Input: part model. Units: mm. Frame: model coordinates. A direction names the side the tool comes from. Coordinates: 2 decimals unless noted, no trailing zeros. Write each loop counter-clockwise with the first axis right and the second up, starting at its lowest first coordinate (ties: lowest second). Pieces come first, ordered by that corner, then holes. Notation, with made-up numbers: (4.5, 54) -> (54.5, 54) arc R21 ccw to (54.5, 63) -> close; hole circle Ø11 at (69.5, 22). An arc over 180 degrees is marked (long way). Use one line per item in the form item = value. Start each with the question number.
(1) Ray query, line 1 along X through (y, z) = (1.5, 0); line 2 along X through (y, z) = (1.5, -55.5); line 3 along Z through (x, y) = (-34.5, 0.5). Return the intervals inside material, ascending.
(2) Cut plane C-C on x = -56. Return the cut outline in (y, z).
(3) First-contact query: pin 1 (1.2 mm diameter, centred on y = 5, z = 0, fed in from +X); pin 2 (2 mm diameter, centred on y = 6, z = -0.5, fed in from -X); pin 3 (1.5 mm diameter, centred on x = -25.5, z = 39.5, fed in from -Y); pin 4 (1.5 mm diameter, centred on y = 9, z = -10, fed in from -X). Flat tips, straight axial feed; report the tip coordinate or a pass-through.
(4) Cut plane D-D on z = -26. Return the cut outline in (x, y) (3 decimals), plus the area to 3 significant figures.
(5) Cut plane B-B on y = 4.75. State how many separate pieces and enclosed holes the cut face has, plus the area to 3 significant figures.
(6) Cut plane A-A on z = -11. Return the cut outline in (x, y) (3 decimals).
(7) Pull-direction query (X, two-part tool) for faces 1 (the face through (62.101, 6, 0)), 2 (the face through (22.38, 4.93, 71.06)), 3 (the face through (-16, 0, 32)); classes: released by +X, released by -X, zero draft, split by the parting line, or undercut.
(8) Set-up query: faces 4 (the face through (65.701, 6, 0)), 5 (the face through (-30.078, 8.479, 51.137)). Return all of +Z, -Z, +X, -X, +Y, -Y with unobstructed straight access to the full face (end or side cutting, diameter ignored); none if empty.
```python
from build123d import *

# Parameters (mm, degrees)
CROQUIS1_R                                     = 74.5
CROQUIS1_R_2                                   = 33
SALIENTE_EXTRUIR1_DEPTH                        = 7
CROQUIS2_R                                     = 74.5
SALIENTE_EXTRUIR2_DEPTH                        = 3
CROQUIS4_R                                     = 2.5
CORTAR_EXTRUIR2_DEPTH                          = 106.832414694
CSK_START                                      = -1
CSK_SLOT_FOR_M3_FLAT_HEAD_MACHINE_SCREW2_DEPTH = 12
CIRPATTERN1_COUNT                              = 6


with BuildPart() as part:
    # Croquis1 → Saliente-Extruir1 (new body)
    with BuildSketch(Plane(origin=(0, 0, 0), x_dir=(1, 0, 0), z_dir=(0, 1, 0))):
        with Locations(Location((0, 0, 0), (0, 0, 270))):
            Circle(CROQUIS1_R)
        with Locations(Location((0, 0, 0), (0, 0, 270))):
            Circle(CROQUIS1_R_2, mode=Mode.SUBTRACT)
    extrude(amount=SALIENTE_EXTRUIR1_DEPTH)

    # Croquis2 → Saliente-Extruir2 (add)
    with BuildSketch(Plane(origin=(0, 7, 0), x_dir=(1, 0, 0), z_dir=(0, 1, 0))):
        with Locations(Location((0, 0, 0), (0, 0, 270))):
            Circle(CROQUIS2_R)
        Polygon((-59.325, 34.25130472), (-59.325, -34.25130472), (0, -68.502609439), (59.325, -34.25130472), (59.325, 34.25130472), (0, 68.502609439), align=None, mode=Mode.SUBTRACT)
    extrude(amount=SALIENTE_EXTRUIR2_DEPTH)

    # Croquis4 → Cortar-Extruir2 (cut, through all)
    with BuildSketch(Plane(origin=(0, 10, 0), x_dir=(1, 0, 0), z_dir=(0, 1, 0))):
        with Locations(Location((17.987923635, 67.131844927, 0), (0, 0, 270))):
            Circle(CROQUIS4_R)
        with Locations(Location((67.131844927, -17.987923635, 0), (0, 0, 270))):
            Circle(CROQUIS4_R)
        with Locations(Location((-17.987923635, -67.131844927, 0), (0, 0, 270))):
            Circle(CROQUIS4_R)
        with Locations(Location((-67.131844927, 17.987923635, 0), (0, 0, 270))):
            Circle(CROQUIS4_R)
    extrude(amount=-CORTAR_EXTRUIR2_DEPTH, mode=Mode.SUBTRACT)

    # CSK SLOT for M3 Flat Head Machine Screw2: read off the stored shape, not the designer's step
    # CSK SLOT for M3 Flat Head Machine Sc 2 → CSK SLOT for M3 Flat Head Machine Screw2 (cut)
    with BuildSketch(Plane(origin=(0, 0, 0), x_dir=(1, 0, 0), z_dir=(0, 1, 0)).offset(CSK_START)):
        with BuildLine():
            ThreePointArc((-31.110894632, -57.903382972), (-28.652048905, -57.244537245), (-29.310894632, -54.785691518))
            Line((-29.310894632, -54.785691518), (-32.774996247, -52.785691518))
            ThreePointArc((-32.774996247, -52.785691518), (-35.233841974, -53.444537245), (-34.574996247, -55.903382972))
            Line((-34.574996247, -55.903382972), (-31.110894632, -57.903382972))
        make_face()
    csk_slot_for_m3_flat_head_machine_screw2 = extrude(amount=CSK_SLOT_FOR_M3_FLAT_HEAD_MACHINE_SCREW2_DEPTH, mode=Mode.SUBTRACT)

    # CSK SLOT for M3 Flat Head Machine Sc 3: loft between two sections, ruled curve by curve
    csk_slot_for_m3_flat_head_machine_sc_3_from = [
        Edge.make_three_point_arc((-29.310894632, 1.35, 54.785691518), (-28.472228144, 1.35, 55.878662964), (-28.652048905, 1.35, 57.244537245)),
        Edge.make_three_point_arc((-28.652048905, 1.35, 57.244537245), (-29.74502035, 1.35, 58.083203732), (-31.110894632, 1.35, 57.903382972)),
        Edge.make_three_point_arc((-34.574996247, 1.35, 55.903382972), (-35.413662734, 1.35, 54.810411526), (-35.233841974, 1.35, 53.444537245)),
        Edge.make_three_point_arc((-35.233841974, 1.35, 53.444537245), (-34.140870528, 1.35, 52.605870758), (-32.774996247, 1.35, 52.785691518)),
        Edge.make_line((-31.110894632, 1.35, 57.903382972), (-34.574996247, 1.35, 55.903382972)),
        Edge.make_line((-29.310894632, 1.35, 54.785691518), (-32.774996247, 1.35, 52.785691518)),
    ]
    csk_slot_for_m3_flat_head_machine_sc_3_to = [
        Edge.make_three_point_arc((-28.635894632, 0, 53.616557223), (-27.168228279, 0, 55.529257253), (-27.48291461, 0, 57.919537245)),
        Edge.make_three_point_arc((-27.48291461, 0, 57.919537245), (-29.39561464, 0, 59.387203598), (-31.785894632, 0, 59.072517267)),
        Edge.make_three_point_arc((-35.249996247, 0, 57.072517267), (-36.7176626, 0, 55.159817237), (-36.402976269, 0, 52.769537245)),
        Edge.make_three_point_arc((-36.402976269, 0, 52.769537245), (-34.490276239, 0, 51.301870892), (-32.099996247, 0, 51.616557223)),
        Edge.make_line((-31.785894632, 0, 59.072517267), (-35.249996247, 0, 57.072517267)),
        Edge.make_line((-28.635894632, 0, 53.616557223), (-32.099996247, 0, 51.616557223)),
    ]
    csk_slot_for_m3_flat_head_machine_sc_3 = Solid(Shell([*[Face.make_surface_from_curves(csk_slot_for_m3_flat_head_machine_sc_3_from[k], csk_slot_for_m3_flat_head_machine_sc_3_to[k]) for k in range(6)], Face(Wire(csk_slot_for_m3_flat_head_machine_sc_3_from)), Face(Wire(csk_slot_for_m3_flat_head_machine_sc_3_to))]))
    add(csk_slot_for_m3_flat_head_machine_sc_3, mode=Mode.SUBTRACT)

    # CirPattern1: CSK SLOT for M3 Flat Head Machine Screw2, CSK SLOT for M3 Flat Head Machine Sc 3 ×6 about axis
    cirpattern1_axis = Axis((0, 0, 0), (0, 1, 0))
    add([csk_slot_for_m3_flat_head_machine_screw2.rotate(cirpattern1_axis, i * 360 / CIRPATTERN1_COUNT) for i in range(1, CIRPATTERN1_COUNT)], mode=Mode.SUBTRACT)
    add([csk_slot_for_m3_flat_head_machine_sc_3.rotate(cirpattern1_axis, i * 360 / CIRPATTERN1_COUNT) for i in range(1, CIRPATTERN1_COUNT)], mode=Mode.SUBTRACT)


solid = part.part
```
Values:
q1.line_1 = -74.5 to -65.7, -62.1 to -33, 33 to 62.1, 65.7 to 74.5
q1.line_2 = -49.7 to -35.06, -28.63 to 28.62, 35.06 to 49.7
q1.line_3 = -66.03 to -56.93, -51.81 to 51.83, 56.93 to 66.03
q2.outline = (0, -49.14) -> (10, -49.14) -> (10, -36.17) -> (7, -36.17) -> (7, 36.17) -> (10, 36.17) -> (10, 49.14) -> (0, 49.14) -> close
q3.pin_1 = 74.5
q3.pin_2 = -74.5
q3.pin_3 = 0
q3.pin_4 = -73.92
q4.outline = (-69.816, 0) -> (-20.322, 0) -> (-20.322, 7) -> (-59.325, 7) -> (-59.325, 10) -> (-69.816, 10) -> close; (20.322, 0) -> (69.816, 0) -> (69.816, 10) -> (59.325, 10) -> (59.325, 7) -> (20.322, 7) -> close
q4.area = 756 mm2
q5.separate_pieces = 1
q5.enclosed_holes = 11
q5.area = 13,800 mm2
q6.outline = (-73.683, 0) -> (-31.113, 0) -> (-31.113, 7) -> (-59.325, 7) -> (-59.325, 10) -> (-73.683, 10) -> close; (31.113, 0) -> (73.683, 0) -> (73.683, 10) -> (59.325, 10) -> (59.325, 7) -> (31.113, 7) -> close
q7.face_1 = undercut
q7.face_2 = split by the parting line
q7.face_3 = zero draft
q8.face_4 = +Y, -Y
q8.face_5 = +Y
